```python
from build123d import *

# Parameters (mm, degrees)
F0_W     = 60
F0_H     = 35
F1_DEPTH = 2
F2_R     = 1.75
F3_DEPTH = 2.001
F4_DEPTH = 10
F5_DEPTH = 10
F6_W     = 80
F6_H     = 36.5470070392
F6_H_2   = 2
F7_DEPTH = 2


with BuildPart() as f1:
    # F0 (on Top) → F1 (new body)
    with BuildSketch(Plane.XY):
        with Locations((30, 17.5)):
            Rectangle(F0_W, F0_H)
    extrude(amount=F1_DEPTH)

    # F2 (on face) → F3 (cut, through all)
    with BuildSketch(Plane.XY.offset(2)):
        with Locations((5, 5)):
            Circle(F2_R)
        with Locations((5, 30)):
            Circle(F2_R)
        with Locations((55, 30)):
            Circle(F2_R)
        with Locations((55, 5)):
            Circle(F2_R)
    extrude(amount=-F3_DEPTH, mode=Mode.SUBTRACT)

    # F4 (add): a face of the model
    f4_faces = [f1.faces().sort_by_distance(p)[0] for p in [
        (60, 17.5, 1),
    ]]
    extrude(f4_faces, amount=F4_DEPTH)

    # F5 (add): a face of the model
    f5_faces = [f1.faces().sort_by_distance(p)[0] for p in [
        (0, 17.5, 1),
    ]]
    extrude(f5_faces, amount=F5_DEPTH)

    # F6 (on face) → F7 (join)
    with BuildSketch(Plane(origin=(0, 35, 0), x_dir=(-1, 0, 0), z_dir=(0, 1, 0))):
        with Locations((-30, -18.2735035196)):
            Rectangle(F6_W, F6_H)
        with Locations((-30, 1)):
            Rectangle(F6_W, F6_H_2)
    extrude(amount=F7_DEPTH)


solid = f1.part
```
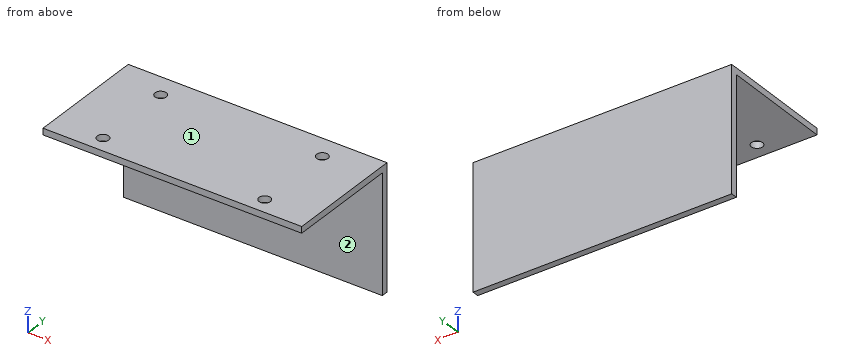
Here's how the part is built. I have some questions about the finished solid (model axes, mm). Face numbers are marked on the shaded views. A direction names the side the tool comes from. Round coordinates to 2 decimals unless told otherwise and drop trailing zeros. Order: outer loops, then holes, each group sorted by start corner. A loop starts at its lowest first (then second) coordinate and runs counter-clockwise, first axis right, second up. Notation, with made-up numbers: M -24.75,-9 L 5.25,-9 A21 cw 5.25,26 Z; hole C -36.75,-23.75 d11. An arc over 180 degrees is marked long. Answer in a Markdown table with one row per item.
Item 1: I'm going to push flat-ended pins straight in: pin 1 (5.5 mm diameter, centred on x = 55, y = 5, fed in from -Z); pin 2 (4 mm diameter, centred on x = 17, z = -26, fed in from -Y); pin 3 (3 mm diameter, centred on x = 5, y = 30, fed in from -Z). Where does each tip first touch, or does it pass through?
A:
| item | result |
|---|---|
| pin 1 | stops at z = 0 |
| pin 2 | stops at y = 35 |
| pin 3 | passes through |
Item 2: Imagine slicing it at B-B, the plane y = 30. Write out the boundary of the cut face in (x, z).
A:
| item | result |
|---|---|
| outline | M -10,0 L 3.25,0 L 3.25,2 L -10,2 Z; M 6.75,0 L 53.25,0 L 53.25,2 L 6.75,2 Z; M 56.75,0 L 70,0 L 70,2 L 56.75,2 Z |
Item 3: If I drill on L1, parallel to Y at x = 55, z = 0.5; L2, parallel to Y at x = 54, z = -11.5; L3, parallel to Z at x = 39, y = 13, over which ranges is the centre line in solid material (lowest first)? Write a range as from..to.
A:
| item | result |
|---|---|
| L1 | y = 0..3.25, 6.75..28.25, 31.75..37 |
| L2 | y = 35..37 |
| L3 | z = 0..2 |
Item 4: Imagine slicing it at D-D, the plane x = 22. Write out the boundary of the cut face in (y, z), and give its area (3 significant figures).
A:
| item | result |
|---|---|
| outline | M 0,0 L 35,0 L 35,-36.55 L 37,-36.55 L 37,2 L 0,2 Z |
| area | 147 mm2 |
Item 5: For the marked faces 1 and 2, which set-ups out of +Z, -Z, +X, -X, +Y, -Y let a thin tool reach every point of the face, with its end or its side?
A:
| item | result |
|---|---|
| face 1 | +Z, +X, -X, +Y, -Y |
| face 2 | -Z, +X, -X, -Y |
Item 6: Imagine slicing it at A-A, the plane x = 55. Write out the boundary of the cut face in (y, z).
A:
| item | result |
|---|---|
| outline | M 0,0 L 3.25,0 L 3.25,2 L 0,2 Z; M 6.75,0 L 28.25,0 L 28.25,2 L 6.75,2 Z; M 31.75,0 L 35,0 L 35,-36.55 L 37,-36.55 L 37,2 L 31.75,2 Z |
Item 7: Imagine slicing it at C-C, the plane z = -14. Write out the boundary of the cut face in (x, y).
A:
| item | result |
|---|---|
| outline | M -10,35 L 70,35 L 70,37 L -10,37 Z |
